```python
from build123d import *

# Parameters (mm, degrees)
CIRPATTERN1_COUNT = 6
SKETCH4_R         = 1.2065


with BuildPart() as part:
    # Sketch1 → Revolve1 (revolve)
    with BuildSketch(Plane.XY, mode=Mode.PRIVATE) as revolve1_sk:
        Polygon((0, 55.8), (1, 55.8), (1, 44.8), (5, 44.8), (5, 42.4), (14, 42.4), (14, 2.4), (5, 2.4), (5, 0), (0, 0), align=None)
    revolve(revolve1_sk.sketch.rotate(Axis((0, 0, 0), (0, 1, 0)), 90), axis=Axis((0, 0, 0), (0, 1, 0)))

    # Sketch2 → M2.5x0.45 Tapped Hole1 (revolve, cut)
    with BuildSketch(Plane(origin=(0, 42.4, -8), x_dir=(0, 0, 1), z_dir=(1, 0, 0))):
        Polygon((0, 0), (0, 4.615874135), (1.025, 3.999992), (1.025, 0), align=None)
    m2_5x0_45_tapped_hole1 = revolve(axis=Axis((0, 48.75, -8), (0, -1, 0)), mode=Mode.SUBTRACT)

    # CirPattern1: M2.5x0.45 Tapped Hole1 ×6 about axis
    cirpattern1_axis = Axis((0, 0, 0), (0, 1, 0))
    for i in range(1, CIRPATTERN1_COUNT):
        add(m2_5x0_45_tapped_hole1.rotate(cirpattern1_axis, i * 360 / CIRPATTERN1_COUNT), mode=Mode.SUBTRACT)

    # Sweep1: sweep along a path in Sketch5
    with BuildLine(Plane(origin=(0, 0, 0), x_dir=(0, 0, -1), z_dir=(1, 0, 0))) as sweep1_path:
        Line((-8, 2.4), (-8, -13.6))
        ThreePointArc((-8, -13.6), (-5.656854249, -19.256854249), (0, -21.6))
        Line((0, -21.6), (8, -21.6))
    # Sketch4 → Sweep1 (sweep)
    with BuildSketch(Plane(origin=(0, 2.4, 0), x_dir=(-1, 0, 0), z_dir=(0, -1, 0))):
        with Locations((-2.507789784, -7.596775)):
            Circle(SKETCH4_R)
        with Locations((0, -8)):
            Circle(SKETCH4_R)
        with Locations((2.507789784, -7.596775)):
            Circle(SKETCH4_R)
    sweep(path=sweep1_path.line)


solid = part.part
```
For this review, take the finished solid that the model builds, in its own axes (mm). A direction names the side the tool comes from. Round coordinates to 2 decimals unless told otherwise and drop trailing zeros. Write each loop counter-clockwise with the first axis right and the second up, starting at its lowest first coordinate (ties: lowest second). Pieces come first, ordered by that corner, then holes. Notation, with made-up numbers: (-6, -6.75) - (50, -6.75) arc R17 cw to (50, 11.25) - close; hole circle Ø4 at (-24.75, 13.25). An arc over 180 degrees is marked (long way). Answer as CSV lines item,"result". Start each with the question number.
(1) Add section D-D, the plane z = -9.75. State the section outline as (x, y) points, plus the area to 3 significant figures.
(2) Add section B-B, the plane x = -2.5. State the section outline as (y, z) points.
(3) Add section C-C, the plane y = 18. State the section outline as (x, z) points, plus the area to 3 significant figures.
(4) For line 1 (Y direction, x = -2.5, z = -2.75); line 2 (X direction, y = 40.6, z = 4); line 3 (Y direction, x = -5.75, z = -1), list the stretches that pass through material, from the lowest coordinate up.
(5) Mouldability with a two-part tool opening along Z and no side actions: class faces 1 (the flat face through (3, -21, -8)), 2 (the cylindrical face through (3.397, -20.381, -4.056)), 3 (the conical face through (6.75, 37.89, 3.98)) as +Z half, -Z half, draft (parallel to the pull), parting line (faces both ways), or undercut.
(6) Machinability: for faces 4 (the flat face through (0, 0, 0)), 5 (the cylindrical face through (3.713, -5.712, 7.544)), 6 (the cylindrical face through (-0.649, -20.583, -4.056)), 7 (the flat face through (0, -22, -8)), 8 (the cylindrical face through (1, 50, 0)), which of the approach directions +Z, -Z, +X, -X, +Y, -Y give a long, thin tool a straight path to every point of the face, cutting with its end or side? Answer none if there is none.
(7) For pin 1 (1.2 mm diameter, centred on x = 0, z = -8, fed in from +Y); pin 2 (1.9 mm diameter, centred on x = 3, y = -21.5, fed in from -Z); pin 3 (1 mm diameter, centred on x = 6.5, y = 6.5, fed in from -Z), all flat-tipped, find the tip position at first contact; note any pin that passes through.
(8) Add section A-A, the plane y = 40.5. State how many separate pieces and enclosed holes the cut face has, plus the area to 3 significant figures.
From the geometry:
1,outline,"(-10.05, 2.4) - (10.05, 2.4) - (10.05, 42.4) - (-10.05, 42.4) - close"
1,area,"804 mm²"
2,outline,"(-22.4, -8) - (-19.99, -8) - (-19.99, 0) arc R6.39 cw to (-13.6, 6.39) - (2.4, 6.39) - (2.4, 4.33) - (0, 4.33) - (0, -4.33) - (2.4, -4.33) - (2.4, -13.77) - (42.4, -13.77) - (42.4, -4.33) - (44.8, -4.33) - (44.8, 4.33) - (42.4, 4.33) - (42.4, 13.77) - (2.4, 13.77) - (2.4, 8.8) - (-13.6, 8.8) arc R8.8 ccw to (-22.4, 0) - close"
3,outline,"circle Ø28 at (0, 0)"
3,area,"616 mm²"
4,line 1,"y = -22.4 to -19.99, 0 to 44.8"
4,line 2,"x = -13.42 to -7.95, -5.9 to 5.9, 7.95 to 13.42"
4,line 3,"y = 2.4 to 42.4"
5,face 1,"-Z half"
5,face 2,"draft"
5,face 3,"undercut"
6,face 4,"-Z, +X, -X"
6,face 5,"none"
6,face 6,"-Z"
6,face 7,"-Z, +X, -X, -Y"
6,face 8,"+Y"
7,pin 1,"stops at y = 38.14"
7,pin 2,"stops at z = -8"
7,pin 3,"stops at z = -12.65"
8,separate pieces,"1"
8,enclosed holes,"6"
8,area,"596 mm²"
